Autodesk Inventor part; units mm, degrees
ref_plane "YZ Plane" through (0, 0, 0) normal (1, 0, 0) x (0, 1, 0)
ref_plane "XZ Plane" through (0, 0, 0) normal (0, 1, 0) x (-1, 0, 0)
ref_plane "XY Plane" through (0, 0, 0) normal (0, 0, 1) x (1, 0, 0)
sketch "Boceto1" plane through (0, 0, 0) normal (0, 1, 0) x (-1, 0, 0)
  line L0 (-52, -2) -> (-52, -55)
  line L1 (-52, -67) -> (0, -67)
  line L2 (0, -67) -> (0, -2)
  line L3 (-52, -2) -> (-40.5, -2)
  line L4 (-40.5, -2) -> (-38, 0)
  line L5 (-38, 0) -> (-4.5, 0)
  line L6 (0, -2) -> (-2, -2)
  line L7 (-4.5, 0) -> (-2, -2)
  line L8 (-52, -67) -> (-52, -55)
  circle A0 centre (-49.4429, -55) radius 2
  circle A1 centre (-2.5817, -53) radius 2
  circle A2 centre (-35.5, -2.2598) radius 2
  line L9 (-4.5, 0) -> (-7, 0)
  circle A3 centre (-5.75, -2.2598) radius 2
  point P0 (0, 0)
extrude "Extrusión1" add sketch "Boceto1" along normal blind 1
sketch "Boceto2" plane through (0, 1, 0) normal (0, 1, 0) x (1, 0, 0)
  line L0 (49, 3) -> (51, 3)
  line L1 (51, 3) -> (51, 50.5)
  line L2 (40.5, 2) -> (52, 2)
  line L3 (52, 2) -> (52, 67)
  line L4 (49, 3) -> (49, 50.5)
  line L5 (49, 50.5) -> (51, 50.5)
  line L6 (1.1059, 3) -> (3, 3)
  line L7 (0, 2) -> (2, 2)
  line L8 (0, 67) -> (0, 2)
  line L9 (1.1059, 3) -> (1, 3)
  line L10 (1, 3) -> (1, 41)
  line L11 (1, 41) -> (3.1059, 41)
  line L12 (3, 41) -> (3, 3)
  point P0 (0, 0)
extrude "Extrusión2" add sketch "Boceto2" along normal blind 8.45
sketch "Boceto3" plane through (0, 1, 0) normal (0, 1, 0) x (1, 0, 0)
  line L0 (30.5, 1) -> (30.5, 5)
  line L1 (24, 1) -> (24, 5)
  line L2 (24, 5) -> (30.5, 5)
  line L3 (30.5, 1) -> (24, 1)
  point P0 (0, 0)
  point P1 (38, 0)
extrude "Extrusión3" add sketch "Boceto3" along normal blind 8
sketch "Boceto4" plane through (0, 1, 0) normal (0, 1, 0) x (1, 0, 0)
  line L0 (42, 67) -> (42, 59.5)
  line L1 (42, 59.5) -> (30, 59.5)
  line L2 (30, 59.5) -> (30, 75.5)
  line L3 (30, 75.5) -> (42, 75.5)
  line L4 (42, 75.5) -> (42, 67)
  point P0 (0, 0)
  point P1 (52, 67)
extrude "Extrusión4" add sketch "Boceto4" along normal blind 10
sketch "Boceto5" plane through (0, 1, 0) normal (0, 1, 0) x (1, 0, 0)
  line L0 (2.5, 67) -> (2.5, 59)
  line L1 (2.5, 59) -> (10.5, 59)
  line L2 (10.5, 59) -> (10.5, 73)
  line L3 (10.5, 73) -> (2.5, 73)
  line L4 (2.5, 73) -> (2.5, 67)
  point P0 (0, 0)
  point P1 (0, 67)
extrude "Extrusión5" add sketch "Boceto5" along normal blind 10
sketch "Boceto6" plane through (2.5, 1, -59) normal (0, 0, 1) x (1, 0, 0)
  line L0 (0, 10) -> (8, 10)
  arc A0 (7.8719, 6) -> (0.1281, 6) centre (4, 6) ccw
  line L1 (8, 0) -> (8, 10)
  line L2 (0, 6) -> (0.1281, 6)
  line L3 (7.8719, 6) -> (8, 6)
  line L4 (8, 6) -> (8, 10)
  line L5 (0, 10) -> (8, 10)
  line L6 (0, 0) -> (0, 10)
  line L7 (0, 10) -> (0, 6)
  point P0 (-2.5, -1)
extrude "Extrusión6" cut sketch "Boceto6" against normal blind 12
sketch "Boceto7" plane through (0, 1, 0) normal (0, 1, 0) x (1, 0, 0)
  line L0 (33.4324, 46.0381) -> (33.4324, 19.5952) construction
  line L1 (33.4324, 19.5952) -> (29.7026, 19.5952) construction
  line L2 (29.7026, 19.5952) -> (29.7026, 46.0381) construction
  line L3 (29.7026, 46.0381) -> (33.4324, 46.0381) construction
equation "\"Radio_pliegue\" = Grosor"
equation "\"Anchura_desahogo_plegado\" = Grosor"
equation "\"Profundidad_desahogo_plegado\" = 0.5 * Grosor"
equation "\"Tamaño_destalonado\" = 4 * Grosor"
equation "\"Remanente_mínimo\" = 2 * Grosor"
equation "\"Radiodetransición\" = Radio_pliegue"
equation "\"Tamaño_de_radio_de_Jacobi\" = Radio_pliegue"
equation "\"TamañoSeparación\" = Grosor"
properties part number "arduino uno"
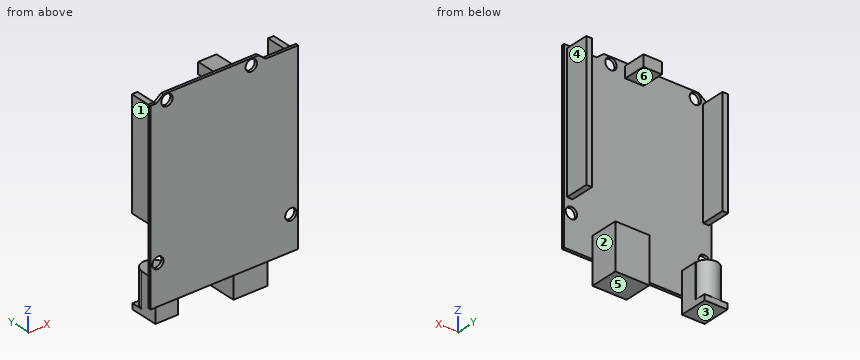
Could you check a few things on this model? Use its own coordinates, in mm. Face numbers are marked on the shaded views. A direction names the side the tool comes from. Give positions to 0.01 mm unless a question says otherwise; leave off trailing zeros. Loops run counter-clockwise (first coordinate to the right, second up) from the corner with the lowest first, then second, coordinate; pieces in that order, holes last. Notation, with made-up numbers: M 84,79 L 113,79 A18 ccw 113,87 Z; hole C 4,20.5 d4. An arc over 180 degrees is marked long. Answer as a JSON object with one key per item and string values.
Q1. For the marked faces 1, 2 and 3, which set-ups out of +Z, -Z, +X, -X, +Y, -Y let a thin tool reach every point of the face, with its end or its side?
Values found:
{"face 1": "+Z, -Z, -X, +Y", "face 2": "+Z, -Z, +X, +Y", "face 3": "-Z, -X, +Y, -Y"}
Q2. Suppose I cut it at A-A, the plane y = 5.5. List the corners of the cut face in (x, z) for me.
Values found:
{"outline": "M 1,-41 L 3,-41 L 3,-3 L 1,-3 Z; M 2.5,-73 L 10.5,-73 L 10.5,-59 L 2.5,-59 Z; M 24,-5 L 30.5,-5 L 30.5,-1 L 24,-1 Z; M 30,-75.5 L 42,-75.5 L 42,-59.5 L 30,-59.5 Z; M 49,-50.5 L 51,-50.5 L 51,-3 L 49,-3 Z"}
Q3. Suppose I cut it at B-B, the plane x = 35.5. List the corners of the cut face in (y, z) for me.
Values found:
{"outline": "M 0,-67 L 1,-67 L 1,-75.5 L 11,-75.5 L 11,-59.5 L 1,-59.5 L 1,-4.26 L 0,-4.26 Z; M 0,-0.26 L 1,-0.26 L 1,0 L 0,0 Z"}
Q4. If I drill on probe 1 along Z at (x, y) = (5.75, 0.65); probe 2 along X at (y, z) = (5.75, -36.5); probe 3 along Z at (x, y) = (31, 10.75), over which ranges is the centre line in solid material (lowest first)? Write a range as [from, to].
Values found:
{"probe 1": "z = [-67, -4.26], [-0.26, 0]", "probe 2": "x = [1, 3], [49, 51]", "probe 3": "z = [-75.5, -59.5]"}
Q5. For P1, Ø1, axis at x = 50, z = -25.5, coming from the +Y side; P2, Ø0.5, axis at x = 48.5, y = 0.5, coming from the +Z side; P3, Ø1.5, axis at x = 42.5, y = 8.5, coming from the +Z side, each with a flat end and sliding along its axis, tell me the tip position at first contact or that it passes through.
Values found:
{"P1": "stops at y = 9.45", "P2": "stops at z = -2", "P3": "stops at z = -59.5"}
Q6. Suppose I cut it at D-D, the plane x = 5.75. List the corners of the cut face in (y, z) for me, plus the area to 3 significant figures.
Values found:
{"outline": "M 0,-67 L 1,-67 L 1,-73 L 11,-73 L 11,-71 L 10.8,-71 L 10.8,-59 L 1,-59 L 1,-4.26 L 0,-4.26 Z; M 0,-0.26 L 1,-0.26 L 1,0 L 0,0 Z", "area": "201 mm²"}
Q7. If we mould it in two halves opening along X, with no side actions, what happens to the marked faces 4, 5 and 6? For each: pulls with the +X half, pulls with the -X half, needs draft (parallel to the pull), parting line crosses it, or undercut.
Values found:
{"face 4": "pulls with the +X half", "face 5": "needs draft", "face 6": "undercut"}
Q8. Suppose I cut it at C-C, the plane z = -63. List the corners of the cut face in (x, y) for me, plus the area to 3 significant figures.
Values found:
{"outline": "M 0,0 L 52,0 L 52,1 L 42,1 L 42,11 L 30,11 L 30,1 L 10.5,1 L 10.5,7 L 10.37,7 A3.87 ccw 2.63,7 L 2.5,7 L 2.5,1 L 0,1 Z", "area": "244 mm²"}
